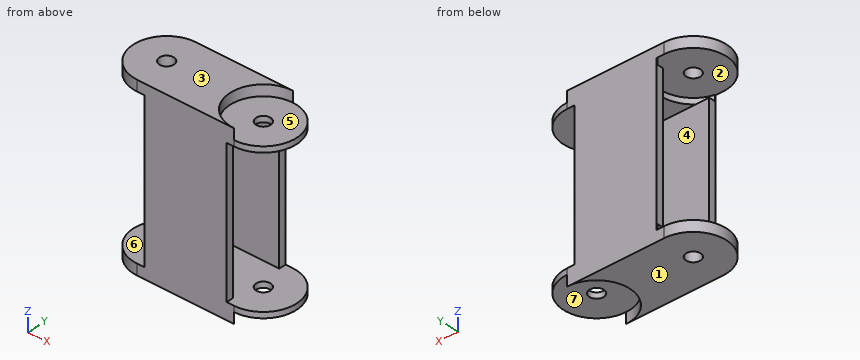
Autodesk Inventor part; units mm, degrees
ref_plane "YZ Plane" through (0, 0, 0) normal (1, 0, 0) x (0, 1, 0)
ref_plane "XZ Plane" through (0, 0, 0) normal (0, 1, 0) x (-1, 0, 0)
ref_plane "XY Plane" through (0, 0, 0) normal (0, 0, 1) x (1, 0, 0)
sketch "Sketch1" plane through (0, 0, 0) normal (0, 0, 1) x (1, 0, 0)
  arc A0 (0, 11.5) -> (0, -11.5) centre (0, 0) ccw
  line L0 (0, 0) -> (-33.5, 0) construction
  line L1 (-33.5, 11.5) -> (0, 11.5)
  line L2 (0, 11.5) -> (0, -11.5)
  line L3 (0, -11.5) -> (-33.5, -11.5)
  line L4 (-33.5, -11.5) -> (-33.5, 11.5)
  line L5 (-31, 9) -> (-2.5, 9)
  line L6 (-2.5, 9) -> (-2.5, -9)
  line L7 (-2.5, -9) -> (-31, -9)
  line L8 (-31, -9) -> (-31, 9)
  arc A1 (-33.5, -11.5) -> (-33.5, 11.5) centre (-33.5, 0) ccw
  arc A2 (-33.5, 11.5) -> (-33.5, -11.5) centre (-33.5, 0) ccw
  arc A3 (0, -11.5) -> (0, 11.5) centre (0, 0) ccw
  line L9 (-31, 9) -> (-31, 11.5)
  line L10 (-2.5, 9) -> (-2.5, 11.5)
  line L11 (-31, -9) -> (-31, -11.5)
  line L12 (-2.5, -9) -> (-2.5, -11.5)
  dimension "d0" = 2.5
  dimension "d1" = 2.5
  dimension "d2" = 2.5
  dimension "d3" = 2.5
  dimension "d4" = 18
  dimension "d5" = 33.5
extrude "Extrusion3" add sketch "Sketch1" along normal mid plane 61.5 contours A0 L10 L1 | A0 L5 A1 L9 L1 L10 | L3 L12 A0 | A0 L7 A1 L5 | L9 A1 L1 | L12 L3 L11 A1 L7 A0 | A1 L7 L8 L5 | L5 L9 A1 | A1 L9 L8 L11 L4 | L4 A2 | L3 A1 L11 | A1 L11 L7
extrude "Extrusion4" add sketch "Sketch1" along normal mid plane 54 contours L2 A0 L12 L6 L10 | A3 L2 | L10 L5 A0 | L5 L6 L7 A0 | A0 L7 L12
extrude "Extrusion5" cut sketch "Sketch1" along normal mid plane 50
extrude "Extrusion7" cut sketch "Sketch1" along normal mid plane 54 contours L9 A1 L1 | A1 L7 L8 L5 | L5 L9 A1 | A1 L9 L8 L11 L4 | L4 A2 | L3 A1 L11 | A1 L11 L7
extrude "Extrusion6" add sketch "Sketch1" along normal mid plane 50 contours L10 L5 A0 | A0 L5 A1 L9 L1 L10 | L12 L3 L11 A1 L7 A0 | A0 L7 L12 | L5 L9 A1 | A1 L11 L7
hole "Hole1" at (-33.5, 0, 0) at (0, 0, 0) direction (0, 0, 1) diameter 5 end through all
hole "Hole2" at (0, 0, 0) at (-33.5, 0, 0) direction (0, 0, -1) diameter 5 end through all
equation "\"d1\" = d0"
equation "\"d2\" = d0"
equation "\"d3\" = d0"
properties part number "carrier-link" material "ABS Plastic"
Check sheet for the modelled part. Datum: model origin and axes. Units: mm. Face numbers are marked on the shaded views. A direction names the side the tool comes from. Give positions to 0.01 mm unless a question says otherwise; leave off trailing zeros. Write each loop counter-clockwise with the first axis right and the second up, starting at its lowest first coordinate (ties: lowest second). Pieces come first, ordered by that corner, then holes. Notation, with made-up numbers: (5.5, 30.5) - (23.5, 30.5) arc R20 cw to (23.5, 49.5) - close; hole circle Ø7 at (39.5, 58). An arc over 180 degrees is marked (long way). Answer as a JSON object with one key per item and string values. Group by question number.
1) Sectioned sample at A-A (x = -15). Record the cut outline in (y, z).
2) Release check for a two-part mould opening along Z. For the marked faces 1, 2 and 3 record: pulls with the +Z half, pulls with the -Z half, needs draft (parallel to the pull), parting line crosses it, or undercut.
3) Access from +Z, -Z, +X, -X, +Y, -Y to the whole of each face (thin tool, end or side, straight path). Record for the marked faces 4, 5, 6 and 7.
4) Sectioned sample at B-B (y = 0). Give the number of separate pieces and of enclosed holes in the cut face, then the cut area to 3 significant figures.
5) Depth check by flat-ended pin: P1, Ø3, axis at y = -10.5, z = -3.5, coming from the -X side; P2, Ø7, axis at x = 1, y = -1, coming from the +Z side; P3, Ø12, axis at y = -1.5, z = 16.5, coming from the +X side; P4, Ø0.8, axis at y = 10.5, z = 10, coming from the +X side. Enter the tip coordinate at first touch or a pass-through.
6) Sectioned sample at D-D (y = 5.25). Record the cut outline in (x, z).
7) Sectioned sample at C-C (x = -1.5). Record the cut outline in (y, z), then the cut area to 3 significant figures.
8) Thickness scan on probe 1 along X at (y, z) = (0, -30); probe 2 along Y at (x, z) = (-21, -12.5); probe 3 along Z at (x, y) = (-23, 7.5). Record the ranges inside material, lowest first. Write a range as from..to.
Geometry results:
{
 "1": {"outline": "(-11.5, -30.75) - (11.5, -30.75) - (11.5, 30.75) - (-11.5, 30.75) - close; hole (-9, -25) - (9, -25) - (9, 25) - (-9, 25) - close"},
 "2": {"face 1": "pulls with the -Z half", "face 2": "undercut", "face 3": "pulls with the +Z half"},
 "3": {"face 4": "+X, -X", "face 5": "+Z, +X", "face 6": "-X", "face 7": "-Z, +X"},
 "4": {"separate pieces": "6", "enclosed holes": "0", "area": "328 mm^2"},
 "5": {"P1": "stops at x = -31", "P2": "stops at z = 27", "P3": "passes through", "P4": "stops at x = -2.5"},
 "6": {"outline": "(-43.73, -30.75) - (-10.23, -30.75) - (-10.23, -27) - (10.23, -27) - (10.23, -25) - (-23.27, -25) - (-23.27, -27) - (-43.73, -27) - close; (-43.73, 27) - (-23.27, 27) - (-23.27, 25) - (10.23, 25) - (10.23, 27) - (-10.23, 27) - (-10.23, 30.75) - (-43.73, 30.75) - close"},
 "7": {"outline": "(-11.5, -30.75) - (-11.4, -30.75) - (-11.4, -27) - (-2, -27) - (-2, -25) - (-11.5, -25) - close; (-11.5, 25) - (-2, 25) - (-2, 27) - (-11.4, 27) - (-11.4, 30.75) - (-11.5, 30.75) - close; (2, -27) - (11.4, -27) - (11.4, -30.75) - (11.5, -30.75) - (11.5, -25) - (2, -25) - close; (2, 25) - (11.5, 25) - (11.5, 30.75) - (11.4, 30.75) - (11.4, 27) - (2, 27) - close", "area": "77.5 mm^2"},
 "8": {"probe 1": "x = -45..-36, -31..-11.5", "probe 2": "y = -11.5..-9, 9..11.5", "probe 3": "z = -30.75..-25, 25..30.75"}
}
